The model under review builds one solid part; all positions refer to its coordinate system, in mm. A direction names the side the tool comes from. Coordinates: 2 decimals unless noted, no trailing zeros. Order: outer loops, then holes, each group sorted by start corner. A loop starts at its lowest first (then second) coordinate and runs counter-clockwise, first axis right, second up. Notation, with made-up numbers: (72, 73.25) -> (129, 73.25) arc R16 ccw to (129, 99.25) -> close; hole circle Ø11 at (6, -25). An arc over 180 degrees is marked (long way). Use one line per item in the form item = value. Start each with the question number.
(1) Mouldability with a two-part tool opening along X and no side actions: class faces 1 (the flat face through (126, 128, 25.4)), 2 (the flat face through (125, 0, 150)), 3 (the flat face through (25.4, 128, 163)), 4 (the flat face through (254, 125, 150)) as +X half, -X half, draft (parallel to the pull), parting line (faces both ways), or undercut.
(2) Wall thickness on line 1 along Y through (x, z) = (95, 145); line 2 along Z through (x, y) = (199, 38): over which ranges is each line inside the solid? List them lowest first.
(3) Take a section at A-A (z = 130). State the section outline as (x, y) points.
(4) For faces 5 (the flat face through (128, 228.6, 163)), 6 (the flat face through (125, 16, 304.8)), list the 3-axis set-ups (+Z, -Z, +X, -X, +Y, -Y) from which the entire face can be reached by the end or side of a thin tool; tool diameter is ignored.
(5) Take a section at B-B (y = 73). State the section outline as (x, z) points, then the cut area to 3 significant figures.
Autodesk Inventor part; units mm, degrees
ref_plane "YZ Plane" through (0, 0, 0) normal (1, 0, 0) x (0, 1, 0)
ref_plane "XZ Plane" through (0, 0, 0) normal (0, 1, 0) x (-1, 0, 0)
ref_plane "XY Plane" through (0, 0, 0) normal (0, 0, 1) x (1, 0, 0)
sketch "Sketch1" plane through (0, 0, 0) normal (0, 0, 1) x (1, 0, 0)
  line L0 (0, 0) -> (254, 0)
  line L1 (254, 0) -> (254, 254)
  line L2 (254, 254) -> (0, 254)
  line L3 (0, 254) -> (0, 0)
  dimension "d0" = 254
  dimension "d1" = 254
extrude "Extrusion1" add sketch "Sketch1" along normal blind 304.8
shell "Shell1" thickness 25.4 removed faces 1 at (169.3333, 84.6667, 304.8)
equation "\"d1\" = d0"
properties part number "Blue truck"
Findings:
q1.face_1 = undercut
q1.face_2 = draft
q1.face_3 = undercut
q1.face_4 = +X half
q2.line_1 = 0 to 25.4, 228.6 to 254
q2.line_2 = 0 to 25.4
q3.outline = (0, 0) -> (254, 0) -> (254, 254) -> (0, 254) -> close; hole (25.4, 25.4) -> (228.6, 25.4) -> (228.6, 228.6) -> (25.4, 228.6) -> close
q4.face_5 = +Z
q4.face_6 = +Z, +X, -X, +Y, -Y
q5.outline = (0, 0) -> (254, 0) -> (254, 304.8) -> (228.6, 304.8) -> (228.6, 25.4) -> (25.4, 25.4) -> (25.4, 304.8) -> (0, 304.8) -> close
q5.area = 20,600 mm²
